The listing builds one solid part. Answer for the finished solid, in the listing's coordinates (mm). Give positions to 0.01 mm unless a question says otherwise; leave off trailing zeros. Write each loop counter-clockwise with the first axis right and the second up, starting at its lowest first coordinate (ties: lowest second). Pieces come first, ordered by that corner, then holes. Notation, with made-up numbers: (-7.75, 22.5) - (39.25, 22.5) arc R34 cw to (39.25, 53.5) - close; hole circle Ø5 at (-39, 82.5). An arc over 180 degrees is marked (long way). Write each question's results on one line, items separated by ' | '. Start each with the question number.
Q1. Find the intervals of material crossed by probe 1 along Y at (x, z) = (-20, 2.75); probe 2 along X at (y, z) = (18, 2.5) (3 decimals); probe 3 along X at (y, z) = (-50, 2), in increasing order.
Q2. Section B-B (x = -13) is taken. Determine the outline of the cut face in (y, z).
Q3. Flat-ended cylindrical pins translate along their axes: pin 1 Ø3 at (y, z) = (-53.5, 4) entering from -X; pin 2 Ø1 at (y, z) = (-45.5, 4) entering from +X. Find the tip coordinate at first contact, or state that the pin passes through.
Q4. Section A-A (z = 3) is taken. Determine the outline of the cut face in (x, y).
Q5. Section C-C (y = -38.5) is taken. Determine the outline of the cut face in (x, z).
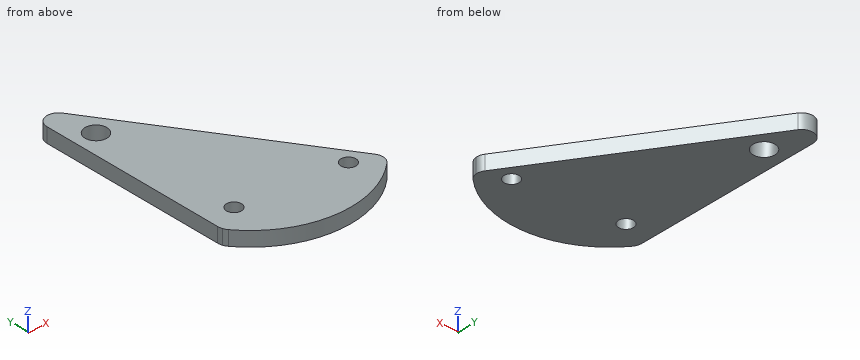
```python
from build123d import *

# Parameters (mm, degrees)
F0_R     = 3.25
F0_R_2   = 4.75
F1_DEPTH = 6.35


# Not quite as in the source:
# - a length typed as a fraction of an inch, garbled in the dataset ("3 / 203.2 mm" for 3/8 in), is restored


with BuildPart() as f1:
    # F0 (on Top) → F1 (new body)
    with BuildSketch(Plane.XY):
        with BuildLine():
            ThreePointArc((-22.8971660057, 33.6711986684), (-28.5061254625, 35.6804376948), (-32.0558722278, 30.8953812108))
            Line((-32.0558722278, 30.8953812108), (-32.0558722278, -50.2885361405))
            ThreePointArc((-32.0558722278, -50.2885361405), (-31.9678509198, -51.3125029104), (-31.7063695792, -52.3064260488))
            Line((-31.7063695792, -52.3064260488), (35.4015681706, -55.732164864))
            ThreePointArc((35.4015681706, -55.732164864), (35.2797878973, -54.0198372397), (34.5860178433, -52.4496208725))
            Line((34.5860178433, -52.4496208725), (-22.8971660057, 33.6711986684))
        make_face()
        with Locations((-20.3956849873, -45.3237444162)):
            Circle(F0_R, mode=Mode.SUBTRACT)
        with Locations((24.9280557036, -50.2885361405)):
            Circle(F0_R, mode=Mode.SUBTRACT)
        with Locations((-22.9451451451, 17.56295003)):
            Circle(F0_R_2, mode=Mode.SUBTRACT)
        with BuildLine():
            Line((35.4015681706, -55.732164864), (-31.7063695792, -52.3064260488))
            ThreePointArc((-31.7063695792, -52.3064260488), (-31.3042287593, -53.1962420607), (-30.763080876, -54.0090450764))
            ThreePointArc((-30.763080876, -54.0090450764), (0.4708891197, -70.6124039736), (33.840882919, -58.8788656243))
            ThreePointArc((33.840882919, -58.8788656243), (34.9066358356, -57.4470716441), (35.4015681706, -55.732164864))
        make_face()
    extrude(amount=F1_DEPTH)


solid = f1.part
```
Answers below:
1) probe 1: y = -63.76 to -48.55, -42.1 to 13.84, 21.29 to 29.33 | probe 2: x = -32.056 to -27.675, -18.215 to -12.437 | probe 3: x = -32.06 to 21.69, 28.17 to 32.95
2) outline: (-67.41, 0) - (18.84, 0) - (18.84, 6.35) - (-67.41, 6.35) - close
3) pin 1: stops at x = -31.81 | pin 2: stops at x = 30.28
4) outline: (-32.06, -50.29) arc R6 ccw to (-30.76, -54.01) arc R44.03 ccw to (33.84, -58.88) arc R5 ccw to (34.59, -52.45) - (-22.9, 33.67) arc R5 ccw to (-32.06, 30.9) - close; hole circle Ø9.5 at (-22.95, 17.56); hole circle Ø6.5 at (-20.4, -45.32); hole circle Ø6.5 at (24.93, -50.29)
5) outline: (-32.06, 0) - (25.28, 0) - (25.28, 6.35) - (-32.06, 6.35) - close
